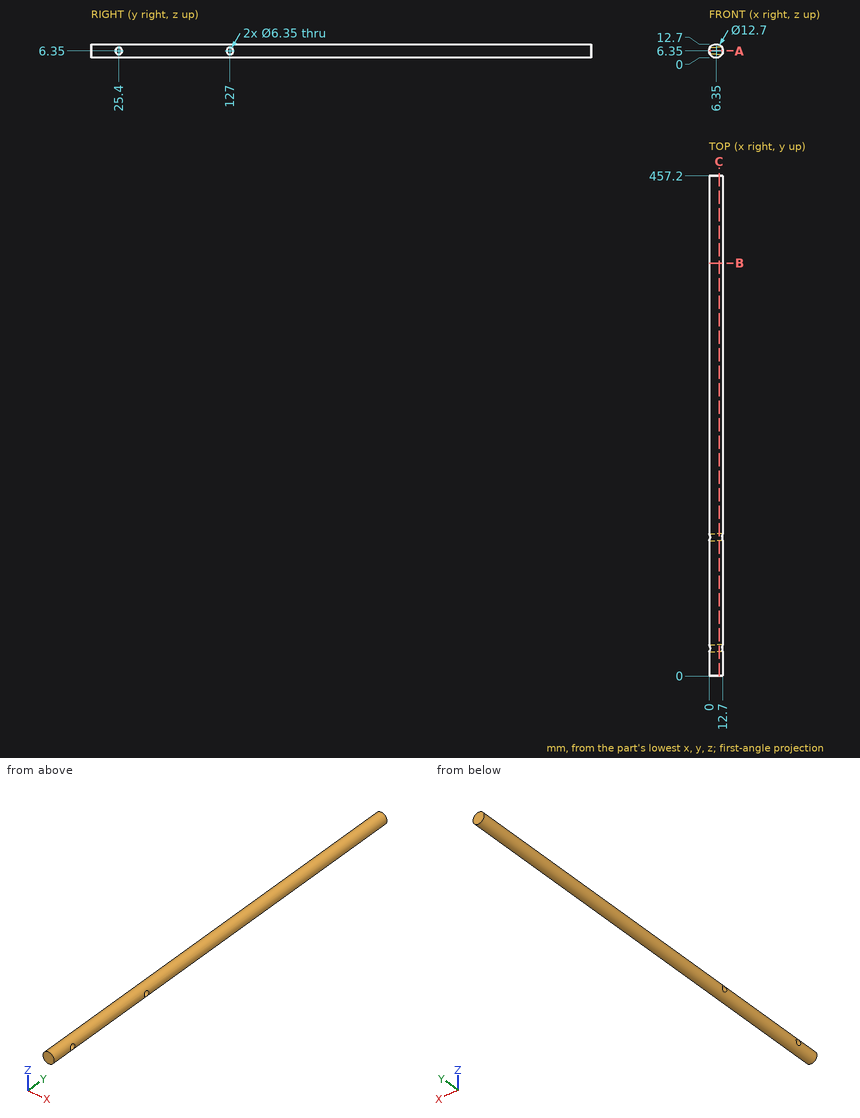
Answer from the drawing. Dimensions are ordinates in mm from the lowest x, y and z of the part. Give positions to 0.01 mm unless a question says otherwise; leave off trailing zeros. Loops run counter-clockwise (first coordinate to the right, second up) from the corner with the lowest first, then second, coordinate; pieces in that order, holes last. Notation, with made-up numbers: (19, 39.5) -> (77, 39.5) arc R20 ccw to (77, 76.5) -> close; hole circle Ø11 at (-5, 14). An arc over 180 degrees is marked (long way). One line per question, with ' | ' between items. Start each with the question number.
1) Section B-B, the plane y = 377.5 is taken. Determine the outline of the cut face in (x, z).
2) Section C-C, the plane x = 9.25 is taken. Determine the outline of the cut face in (y, z) (3 decimals), then the cut area to 3 significant figures.
3) Each of these flat-tipped pins is pushed along its axis until it touches: pin 1 (1 mm diameter, centred on y = 372.5, z = 7, fed in from +X); pin 2 (1.5 mm diameter, centred on x = 4.5, y = 122.5, fed in from +Z). Where does it stop, or does it pass through?
4) Straight lines are drawn through the part: L1, parallel to Y at x = 4.5, z = 6.5; L2, parallel to Y at x = 9.5, z = 9; L3, parallel to X at y = 29, z = 7. For each, find the intervals that lie inside material, in ascending order.
5) Section A-A, the plane z = 6.35 is taken. Determine the outline of the cut face in (x, y) (3 decimals).
Resolved:
1) outline: circle Ø12.7 at (6.35, 6.35)
2) outline: (0, 0.701) -> (457.2, 0.701) -> (457.2, 11.999) -> (0, 11.999) -> close; hole circle Ø6.35 at (25.4, 6.35); hole circle Ø6.35 at (127, 6.35) | area: 5,100 mm2
3) pin 1: x = 12.7 | pin 2: z = 12.6
4) L1: 0 to 22.23, 28.57 to 123.83, 130.17 to 457.2 | L2: 0 to 23.65, 27.15 to 125.25, 128.75 to 457.2 | L3: 0.03 to 12.67
5) outline: (0, 0) -> (12.7, 0) -> (12.7, 22.225) -> (0, 22.225) -> close; (0, 28.575) -> (12.7, 28.575) -> (12.7, 123.825) -> (0, 123.825) -> close; (0, 130.175) -> (12.7, 130.175) -> (12.7, 457.2) -> (0, 457.2) -> close
